from build123d import *

# Parameters (mm, degrees)
FILLET1_R      = 0.25
CHAMFER1_SIZE  = 0.5
CHAMFER1_SIZE2 = 0.288675135
CHAMFER2_SIZE  = 0.5


with BuildPart() as part:
    # Sketch1 → Revolve1 (revolve)
    with BuildSketch(Plane.XY):
        Polygon((1.85, 0), (1.85, -4.5), (1.5, -4.5), (1.5, -9.8), (2.45, -9.8), (2.45, -0.75), (3.95, -0.75), (3.95, 0), align=None)
    revolve(axis=Axis((0, 0, 0), (0, -1, 0)))

    # Fillet1
    fillet1_edges = [part.edges().sort_by_distance(p)[0] for p in [
        (-3.95, 0, 0),
        (-3.95, -0.75, 0),
        (-1.85, 0, 0),
    ]]
    fillet(fillet1_edges, radius=FILLET1_R)

    # Chamfer1
    chamfer1_edges = [part.edges().sort_by_distance(p)[0] for p in [
        (-2.45, -9.8, 0),
    ]]
    chamfer1_side = [part.faces().sort_by_distance(p)[0] for p in [
        (-2.45, -5.275, 0),
    ]]
    chamfer(chamfer1_edges, length=CHAMFER1_SIZE, length2=CHAMFER1_SIZE2, reference=chamfer1_side[0])

    # Chamfer2
    chamfer2_edges = [part.edges().sort_by_distance(p)[0] for p in [
        (-1.5, -9.8, 0),
    ]]
    chamfer(chamfer2_edges, length=CHAMFER2_SIZE)


solid = part.part
The listing builds one solid part. Answer for the finished solid, in the listing's coordinates (mm). Give positions to 0.01 mm unless a question says otherwise; leave off trailing zeros. Write each loop counter-clockwise with the first axis right and the second up, starting at its lowest first coordinate (ties: lowest second). Pieces come first, ordered by that corner, then holes.
Item 1: Determine the mould class of faces 1 (the cylindrical face through (-0.5, -5, -2.4)), 2 (the cylindrical face through (-0.401, -2.405, -1.806)), 3 (the flat face through (0, -0.75, 3)), 4 (the cylindrical face through (-1.5, -6.93, 0.07)) for opening direction X: released by +X, released by -X, zero draft, split by the parting line, or undercut.
Item 2: Section A-A, the plane x = 0 is taken. Write down the section's boundary in (y, z).
Item 3: Section B-B, the plane y = -7.5 is taken. Write down the section's boundary in (x, z), plus the area to 3 significant figures.
Item 4: Flat-ended cylindrical pins translate along their axes: P1, Ø3, axis at y = -3.5, z = 3, coming from the +X side; P2, Ø4, axis at y = -3.5, z = 2, coming from the +X side; P3, Ø2, axis at x = 2, z = 2, coming from the +Y side; P4, Ø2, axis at x = 0.5, z = -0.5, coming from the +Y side. Find the tip coordinate at first contact, or state that the pin passes through.
Item 5: Find the intervals of material crossed by line 1 along Z through (x, y) = (0, -2.3); line 2 along Z through (x, y) = (0, -7.4); line 3 along Y through (x, z) = (-1.5, 2), in increasing order.
Item 6: Section C-C, the plane y = -1.25 is taken. Write down the section's boundary in (x, z).
Completed:
1. face 1: split by the parting line
1. face 2: undercut
1. face 3: zero draft
1. face 4: undercut
2. outline: (-9.8, -2.16) - (-9.3, -2.45) - (-0.75, -2.45) - (-0.75, -3.7) arc R0.25 ccw to (-0.5, -3.95) - (-0.25, -3.95) arc R0.25 ccw to (0, -3.7) - (0, -2.1) arc R0.25 ccw to (-0.25, -1.85) - (-4.5, -1.85) - (-4.5, -1.5) - (-9.3, -1.5) - (-9.8, -2) - close; (-9.8, 2) - (-9.3, 1.5) - (-4.5, 1.5) - (-4.5, 1.85) - (-0.25, 1.85) arc R0.25 ccw to (0, 2.1) - (0, 3.7) arc R0.25 ccw to (-0.25, 3.95) - (-0.5, 3.95) arc R0.25 ccw to (-0.75, 3.7) - (-0.75, 2.45) - (-9.3, 2.45) - (-9.8, 2.16) - close
3. outline: circle Ø4.9 at (0, 0); hole circle Ø3 at (0, 0)
3. area: 11.8 mm2
4. P1: stops at x = 1.94
4. P2: stops at x = 2.45
4. P3: stops at y = 0
4. P4: stops at y = -4.5
5. line 1: z = -2.45 to -1.85, 1.85 to 2.45
5. line 2: z = -2.45 to -1.5, 1.5 to 2.45
5. line 3: y = -0.75 to 0
6. outline: circle Ø4.9 at (0, 0); hole circle Ø3.7 at (0, 0)
